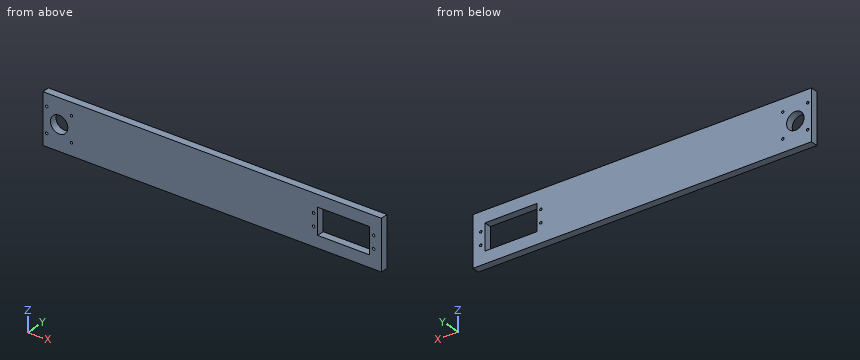
Autodesk Inventor part; units mm, degrees
ref_plane "YZ Plane" through (0, 0, 0) normal (1, 0, 0) x (0, 1, 0)
ref_plane "XZ Plane" through (0, 0, 0) normal (0, 1, 0) x (-1, 0, 0)
ref_plane "XY Plane" through (0, 0, 0) normal (0, 0, 1) x (1, 0, 0)
sketch "Sketch1" plane through (0, 0, 0) normal (0, 1, 0) x (-1, 0, 0)
  line L0 (0, 0) -> (31.5, 0)
  line L1 (0, 0) -> (18.5, 0) construction
  line L2 (0, 0) -> (-10.5, 0)
  line L3 (-20, 0) -> (-20, 20)
  line L4 (-20, 20) -> (253, 20)
  line L5 (253, 20) -> (253, 0)
  line L6 (-10.5, 10.5) -> (31.5, 10.5)
  line L7 (31.5, 10.5) -> (31.5, -10.5)
  line L8 (31.5, -10.5) -> (-10.5, -10.5)
  line L9 (-10.5, -10.5) -> (-10.5, 10.5)
  line L10 (-10.5, 10.5) -> (31.5, -10.5) construction
  line L11 (31.5, 10.5) -> (-10.5, -10.5) construction
  line L12 (-13.75, 5) -> (34.75, 5) construction
  line L13 (34.75, 5) -> (34.75, -5) construction
  line L14 (34.75, -5) -> (-13.75, -5) construction
  line L15 (-13.75, -5) -> (-13.75, 5) construction
  line L16 (-13.75, 5) -> (34.75, -5) construction
  line L17 (34.75, 5) -> (-13.75, -5) construction
  line L18 (31.5, 0) -> (253, 0)
  line L19 (-10.5, 0) -> (-20, 0)
  line L20 (-20, 0) -> (0, 0) construction
  line L21 (240, 0) -> (240, 10) construction
  line L22 (240, 10) -> (250, 10) construction
  point P0 (10.5, 0)
  point P1 (10.5, 0)
  dimension "d28" = 18.5
  dimension "d37" = 20
  dimension "d38" = 20
  dimension "d39" = 42
  dimension "d40" = 21
  dimension "d41" = 48.5
  dimension "d42" = 10
  dimension "d43" = 10.5
  dimension "d52" = 240
  dimension "d53" = 13
  dimension "d54" = 9.5
  dimension "d62" = 10
extrude "Extrusion1" add sketch "Sketch1" along normal blind 6 contours L7 L6 L9 L19 L3 L4 L5 L18
hole "Hole3" at (0, 0, 0) at (13.75, 0, 5) at (-34.75, 0, 5) direction (0, 1, 0) diameter 2 end through all
fillet "Fillet1" [suppressed]
mirror "Mirror1" about plane through (-31.5, 0, 0) normal (0, 0, -1)
hole "Hole4" at (-240, 0, 0) direction (0, 1, 0) diameter 14 end through all
hole "Hole5" at (-250, 0, 10) direction (0, 1, 0) diameter 2 end through all
pattern_circular "Circular Pattern1" count 4 over 360 about axis through (-240, 275.9801, 0) along (0, 1, 0) of "Hole5"
properties part number "segment2b" material "Plywood, Finish"
Can you work these out from the model? Positions are in its coordinate system, mm. Coordinates: 2 decimals unless noted, no trailing zeros. Loops run counter-clockwise (first coordinate to the right, second up) from the corner with the lowest first, then second, coordinate; pieces in that order, holes last. Notation, with made-up numbers: M -13.5,51 L 12.5,51 A22 ccw 12.5,80 Z; hole C 35.5,88 d2. An arc over 180 degrees is marked long. Return JSON: item names as keys, results as strings. Group by question number.
Item 1: Imagine slicing it at B-B (y = 1.1). Give the number of separate pieces and of enclosed holes in the cut face, and give its area (3 significant figures).
Item 2: Imagine slicing it at A-A (z = 0). Please give me the cut outline in (x, y).
Item 3: Imagine slicing it at C-C (x = -240). Please give me the cut outline in (y, z), and give its area (3 significant figures).
Item 4: If I drill on L1, parallel to X at y = 3.2, z = 0.5; L2, parallel to X at y = 1.5, z = -10; L3, parallel to Z at x = -34.75, y = 4.55, over which ranges is the centre line in solid material (lowest first)? Write a range as from..to.
Item 5: I'm going to push a flat-ended pin straight in: pin 1 Ø1.6 at (x, z) = (13.75, 5) entering from -Y. Where does the tip first touch, or does it pass through?
Verdict:
{
 "1": {"separate pieces": "1", "enclosed holes": "10", "area": "9,860 mm^2"},
 "2": {"outline": "M -253,0 L -247,0 L -247,6 L -253,6 Z; M -233,0 L -31.5,0 L -31.5,6 L -233,6 Z; M 10.5,0 L 20,0 L 20,6 L 10.5,6 Z"},
 "3": {"outline": "M 0,-20 L 6,-20 L 6,-7 L 0,-7 Z; M 0,7 L 6,7 L 6,20 L 0,20 Z", "area": "156 mm^2"},
 "4": {"L1": "x = -253..-246.98, -233.02..-31.5, 10.5..20", "L2": "x = -253..-251, -249..-231, -229..-31.5, 10.5..20", "L3": "z = -20..-6, -4..4, 6..20"},
 "5": {"pin 1": "passes through"}
}
